Source: three-view drawing plus pictorial views. Frame: mm from the lowest corner of the part. A direction names the side the tool comes from. Give positions to 0.01 mm unless a question says otherwise; leave off trailing zeros. Loops run counter-clockwise (first coordinate to the right, second up) from the corner with the lowest first, then second, coordinate; pieces in that order, holes last. Notation, with made-up numbers: (72, -5) -> (88, -5) arc R17 cw to (88, 2) -> close; hole circle Ø6 at (30.5, 53.25). An arc over 180 degrees is marked (long way). Answer as a JSON object with one key per item and string values. Group by question number.
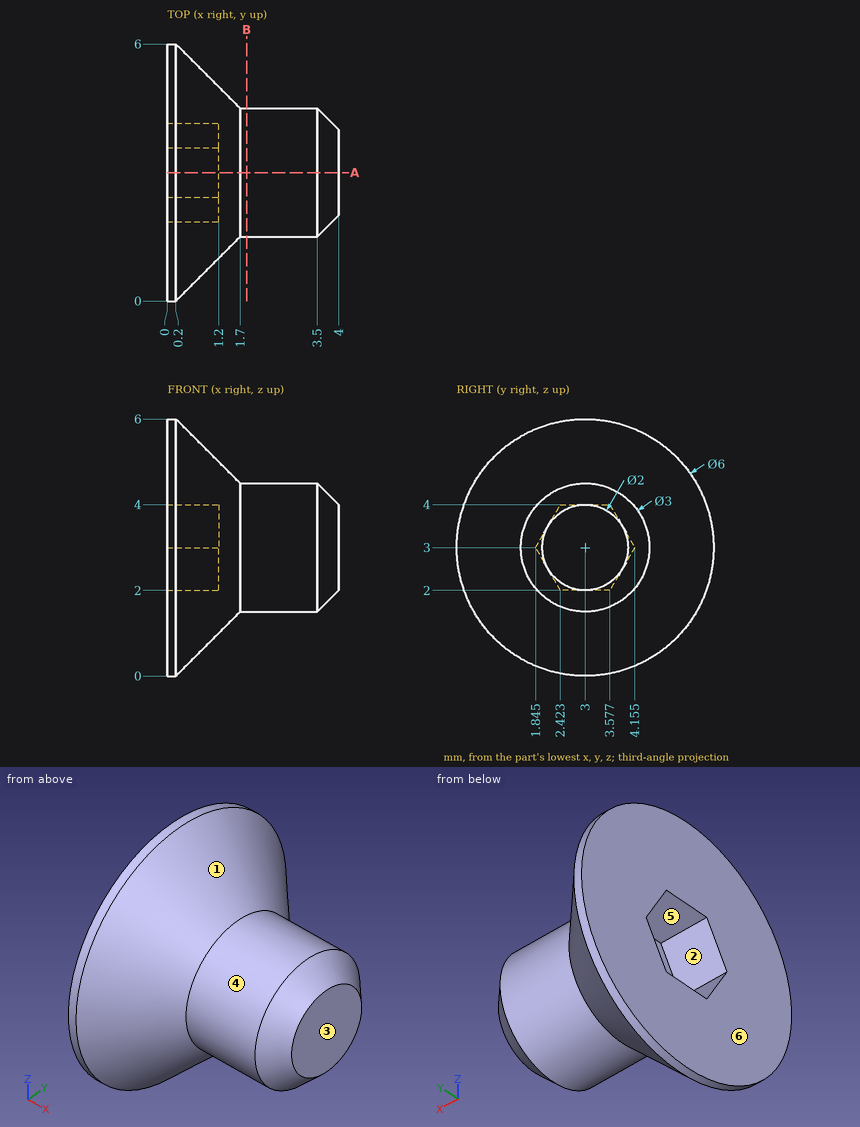
Q1. Section A-A on y = 3. Return the cut outline in (x, z), then the cut area to 3 significant figures.
Q2. Pull-direction query (Z, two-part tool) for the marked faces 1, 2 and 3; classes: +Z half, -Z half, draft (parallel to the pull), parting line (faces both ways), or undercut.
Q3. Ray query, probe 1 along X at (y, z) = (2.85, 3.55); probe 2 along Y at (x, z) = (3.6, 2.25); probe 3 along Y at (x, z) = (2.95, 2.7). Return the intervals inside material, ascending.
Q4. Set-up query: the marked faces 4, 5 and 6. Return all of +Z, -Z, +X, -X, +Y, -Y with unobstructed straight access to the full face (end or side cutting, diameter ignored); none if empty.
Q5. Section B-B on x = 1.85. Return the cut outline in (y, z).
Numbers:
{
 "1": {"outline": "(0, 0) -> (0.2, 0) -> (1.7, 1.5) -> (3.5, 1.5) -> (4, 2) -> (4, 4) -> (3.5, 4.5) -> (1.7, 4.5) -> (0.2, 6) -> (0, 6) -> (0, 4) -> (1.2, 4) -> (1.2, 2) -> (0, 2) -> close", "area": "12.2 mm²"},
 "2": {"face 1": "parting line", "face 2": "undercut", "face 3": "draft"},
 "3": {"probe 1": "x = 1.2 to 4", "probe 2": "y = 1.82 to 4.18", "probe 3": "y = 1.53 to 4.47"},
 "4": {"face 4": "+X", "face 5": "-X", "face 6": "+Z, -Z, -X, +Y, -Y"},
 "5": {"outline": "circle Ø3 at (3, 3)"}
}
